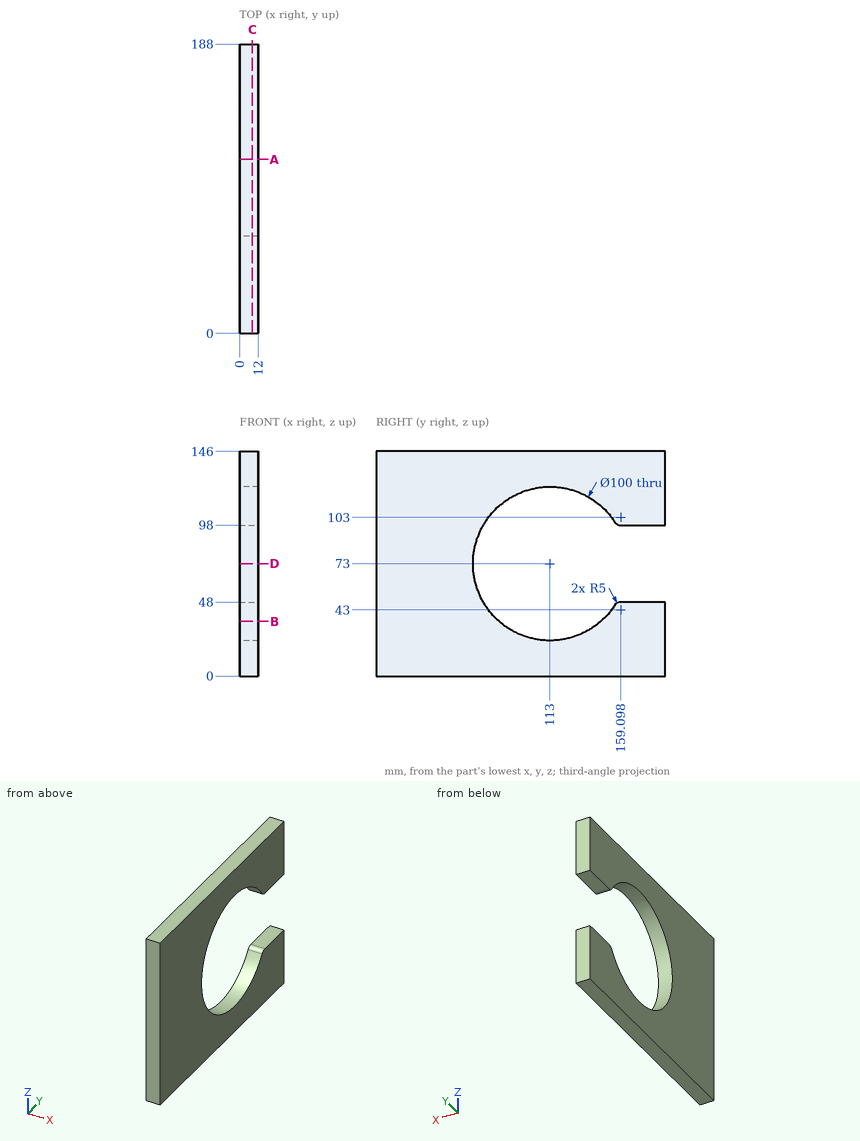
The figure shows three views and two pictorial views of one solid part (mm, origin at its lowest corner). Answer the questions. Coordinates: 2 decimals unless noted, no trailing zeros. Write each loop counter-clockwise with the first axis right and the second up, starting at its lowest first coordinate (ties: lowest second). Pieces come first, ordered by that corner, then holes.
1. A flat-ended cylindrical pin translates along its axis: pin 1 (1 mm diameter, centred on y = 66, z = 85, fed in from -X). Find the tip coordinate at first contact, or state that the pin passes through.
Results list:
pin 1: passes through
2. The part is cut by section A-A, the plane y = 113. Write down the section's boundary in (x, z).
Results list:
outline: (0, 0) - (12, 0) - (12, 23) - (0, 23) - close; (0, 123) - (12, 123) - (12, 146) - (0, 146) - close
3. The part is cut by section C-C, the plane x = 8.25. Write down the section's boundary in (y, z), and give its area (3 significant figures).
Results list:
outline: (0, 0) - (188, 0) - (188, 48) - (159.1, 48) arc R5 ccw to (154.91, 45.73) arc R50 cw (long way) to (154.91, 100.27) arc R5 ccw to (159.1, 98) - (188, 98) - (188, 146) - (0, 146) - close
area: 18,200 mm2
4. The part is cut by section B-B, the plane z = 35.5. Write down the section's boundary in (x, y).
Results list:
outline: (0, 0) - (12, 0) - (12, 79.93) - (0, 79.93) - close; (0, 146.07) - (12, 146.07) - (12, 188) - (0, 188) - close
5. The part is cut by section D-D, the plane z = 73. Write down the section's boundary in (x, y), and give its area (3 significant figures).
Results list:
outline: (0, 0) - (12, 0) - (12, 63) - (0, 63) - close
area: 756 mm2
6. Consider line 1 along Z through (x, y) = (8.25, 113); line 2 along Z through (x, y) = (5.5, 159.5); line 3 along Y through (x, z) = (8.5, 73). Determine where each line is inside the solid, lowest interval first.
Results list:
line 1: z = 0 to 23, 123 to 146
line 2: z = 0 to 48, 98 to 146
line 3: y = 0 to 63
